Can you work these out from the model? Positions are in its coordinate system, mm. Face numbers are marked on the shaded views. A direction names the side the tool comes from. Give positions to 0.01 mm unless a question says otherwise; leave off trailing zeros. Loops run counter-clockwise (first coordinate to the right, second up) from the corner with the lowest first, then second, coordinate; pieces in that order, holes last. Notation, with made-up numbers: (-17.75, -27.75) - (-7.75, -27.75) arc R15 cw to (-7.75, -1.75) - close; hole circle Ø9 at (69, 66). An arc over 180 degrees is marked (long way). Use a Markdown table: item, result. Add a question column.
```python
from build123d import *

# Parameters (mm, degrees)
F0_W          = 25
F0_H          = 10
F1_DEPTH      = 4
F2_W          = 5
F2_H          = 10
F3_DEPTH      = 10
F4_R          = 1.25
F5_DEPTH      = 4.001
F7_R          = 4.99999
F8_R          = 1.55
F9_DEPTH      = 15.001
F10_R         = 1
F11_T1_DEPTH  = 8
F11_T6_ANGLE  = 233.2969892374
F11_T11_ANGLE = 233.2969892374
F11_T16_ANGLE = 233.2969892374
F11_T21_ANGLE = 233.2969892374


# Not quite as in the source:
# - a fillet or chamfer that OpenCascade refuses, or shapes differently, is made with other operations: its cross-section is extruded or revolved along the edge and cut away or added
# - a fillet or chamfer is up to 0.001 mm smaller than in the source, because OpenCascade refuses the exact size
# - a pattern or mirror of a feature is missing from the dataset's text; its kind, count and spacing are read off the source's solid


with BuildPart() as f1:
    # F0 (on Top) → F1 (new body)
    with BuildSketch(Plane.XY):
        Rectangle(F0_W, F0_H)
    extrude(amount=F1_DEPTH)

    # F2 (on face) → F3 (join)
    with BuildSketch(Plane.XY.offset(4)):
        Rectangle(F2_W, F2_H)
    extrude(amount=F3_DEPTH)

    # F4 (on face) → F5 (cut, through all)
    with BuildSketch(Plane.XY.offset(4)):
        with Locations((-7.5, 0)):
            Circle(F4_R)
    f5 = extrude(amount=-F5_DEPTH, mode=Mode.SUBTRACT)

    # F5_copies: F5 across plane
    add(f5.mirror(Plane(origin=(0, 0, 0), x_dir=(0, 0, 1), z_dir=(1, 0, 0))), mode=Mode.SUBTRACT)

    # F7 (radius 5 in the source; OpenCascade refuses exactly that, so slightly less here)
    f7_edges = [f1.edges().sort_by_distance(p)[0] for p in [
        (0, -5, 14),
        (0, 5, 14),
    ]]
    fillet(f7_edges, radius=F7_R)

    # F8 (on face) → F9 (cut, through all)
    with BuildSketch(Plane(origin=(-2.5, 0, 0), x_dir=(0, -1, 0), z_dir=(-1, 0, 0))):
        with Locations((0, 9)):
            Circle(F8_R)
    extrude(amount=-F9_DEPTH, mode=Mode.SUBTRACT)

    # F10
    f10_edges = [f1.edges().sort_by_distance(p)[0] for p in [
        (7.5, -5, 4),
        (12.5, 0, 4),
        (7.5, 5, 4),
        (12.5, -5, 2),
        (12.5, 5, 2),
        (-12.5, -5, 2),
        (-12.5, 5, 2),
        (-12.5, 0, 4),
        (-7.5, -5, 4),
        (-7.5, 5, 4),
    ]]
    fillet(f10_edges, radius=F10_R)

    # F11: fillet of radius 1 on 2 edges, made by hand

    # F11_s2 → F11_t1 (join)
    with BuildSketch(Plane.XZ.offset(-4)):
        with BuildLine():
            ThreePointArc((2.5, 5), (2.7928932188, 4.2928932188), (3.5, 4))
            Line((3.5, 4), (2.5, 4))
            Line((2.5, 4), (2.5, 5))
        make_face()
        with BuildLine():
            ThreePointArc((-2.5, 5), (-2.7928932188, 4.2928932188), (-3.5, 4))
            Line((-3.5, 4), (-2.5, 4))
            Line((-2.5, 4), (-2.5, 5))
        make_face()
    extrude(amount=F11_T1_DEPTH)


with BuildPart() as f11_tool4:
    # F11_s5 → F11_t6 (revolve)
    with BuildSketch(Plane.XZ.offset(-4)):
        with BuildLine():
            ThreePointArc((-2.5, 5), (-2.7928932188, 4.2928932188), (-3.5, 4))
            Line((-3.5, 4), (-2.5, 4))
            Line((-2.5, 4), (-2.5, 5))
        make_face()
    revolve(axis=Axis((-2.5, 4, 3), (-1, 0, 0)), revolution_arc=F11_T6_ANGLE)

    split(bisect_by=Plane.XZ.offset(-5), keep=Keep.TOP)


with BuildPart() as f1_1:
    add(f1.part)

    # F11_t3: union F11_tool4
    add(f11_tool4.part)


with BuildPart() as f11_tool9:
    # F11_s10 → F11_t11 (revolve)
    with BuildSketch(Plane(origin=(0, 0.0087041916, 0.0116762883), x_dir=(1, 0, 0), z_dir=(0, 0.5976672776, 0.8017442393))):
        with BuildLine():
            ThreePointArc((-3.5, -3.9999787901), (-2.7928932188, -3.7070855713), (-2.5, -2.9999787901))
            Line((-2.5, -2.9999787901), (-2.5, -3.9999787901))
            Line((-2.5, -3.9999787901), (-3.5, -3.9999787901))
        make_face()
    revolve(axis=Axis((-2.5, -4, 3), (-1, 0, 0)), revolution_arc=F11_T11_ANGLE)

    split(bisect_by=Plane.XZ.offset(5), keep=Keep.BOTTOM)


with BuildPart() as f1_2:
    add(f1_1.part)

    # F11_t8: union F11_tool9
    add(f11_tool9.part)


with BuildPart() as f11_tool14:
    # F11_s15 → F11_t16 (revolve)
    with BuildSketch(Plane(origin=(0, 0.0087041916, 0.0116762883), x_dir=(1, 0, 0), z_dir=(0, 0.5976672776, 0.8017442393))):
        with BuildLine():
            ThreePointArc((3.5, -3.9999787901), (2.7928932188, -3.7070855713), (2.5, -2.9999787901))
            Line((2.5, -2.9999787901), (2.5, -3.9999787901))
            Line((2.5, -3.9999787901), (3.5, -3.9999787901))
        make_face()
    revolve(axis=Axis((2.5, -4, 3), (-1, 0, 0)), revolution_arc=F11_T16_ANGLE)

    split(bisect_by=Plane.XZ.offset(5), keep=Keep.BOTTOM)


with BuildPart() as f1_3:
    add(f1_2.part)

    # F11_t13: union F11_tool14
    add(f11_tool14.part)


with BuildPart() as f11_tool19:
    # F11_s20 → F11_t21 (revolve)
    with BuildSketch(Plane.XZ.offset(-4)):
        with BuildLine():
            ThreePointArc((2.5, 5), (2.7928932188, 4.2928932188), (3.5, 4))
            Line((3.5, 4), (2.5, 4))
            Line((2.5, 4), (2.5, 5))
        make_face()
    revolve(axis=Axis((2.5, 4, 3), (-1, 0, 0)), revolution_arc=F11_T21_ANGLE)

    split(bisect_by=Plane.XZ.offset(-5), keep=Keep.TOP)


with BuildPart() as f1_4:
    add(f1_3.part)

    # F11_t18: union F11_tool19
    add(f11_tool19.part)


solid = f1_4.part
```
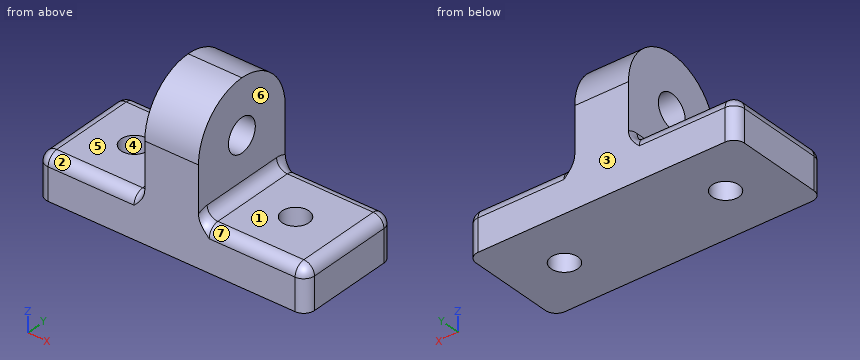
1. Will these pins go through, and if not, where does the flat tip stop? P1, Ø1.9, axis at y = 0, z = 9, coming from the -X side; P2, Ø3, axis at y = -2, z = 9.5, coming from the +X side; P3, Ø3, axis at x = 3.5, y = -2, coming from the +Z side; P4, Ø4, axis at x = -7.5, y = 0, coming from the +Z side.
2. If we mould it in two halves opening along Y, with no side actions, what happens to the marked faces 1, 2, 3 and 4? For each: released by +Y, released by -Y, zero draft, split by the parting line, or undercut.
3. Suppose I cut it at B-B (z = 7.75). List the corners of the cut face in (x, y) for me, and give its area (3 significant figures).
4. Please list where these lines run through material, in increasing order: line 1 along Z through (x, y) = (-0.95, 0); line 2 along Z through (x, y) = (-10.25, 0.75); line 3 along X through (y, z) = (1, 11.75). Write a range as [from, to].
5. Suppose I cut it at D-D (z = 2.5). List the corners of the cut face in (x, y) for me.
6. Suppose I cut it at C-C (x = 7.5). List the corners of the cut face in (y, z) for me, and give its area (3 significant figures).
7. On a 3-axis mill with a long thin cutter (end or side, diameter ignored), from which of +Z, -Z, +X, -X, +Y, -Y can I reach the whole of each face in a straight line? I mean the marked faces 5, 6 and 7. Say none if no direction works.
Results below:
| question | item | result |
|---|---|---|
| 1 | P1 | through |
| 1 | P2 | x = 2.5 |
| 1 | P3 | z = 13.92 |
| 1 | P4 | z = 4 |
| 2 | face 1 | zero draft |
| 2 | face 2 | released by -Y |
| 2 | face 3 | released by +Y |
| 2 | face 4 | undercut |
| 3 | outline | (-2.5, -5) - (2.5, -5) - (2.5, -0.92) - (-2.5, -0.92) - close; (-2.5, 0.92) - (2.5, 0.92) - (2.5, 5) - (-2.5, 5) - close |
| 3 | area | 40.8 mm² |
| 4 | line 1 | [0, 7.45], [10.55, 14] |
| 4 | line 2 | [0, 4] |
| 4 | line 3 | [-2.5, 2.5] |
| 5 | outline | (-12.5, -4) arc R1 ccw to (-11.5, -5) - (11.5, -5) arc R1 ccw to (12.5, -4) - (12.5, 4) arc R1 ccw to (11.5, 5) - (-11.5, 5) arc R1 ccw to (-12.5, 4) - close; hole circle Ø2.5 at (-7.5, 0); hole circle Ø2.5 at (7.5, 0) |
| 6 | outline | (-5, 0) - (-1.25, 0) - (-1.25, 4) - (-4, 4) arc R1 ccw to (-5, 3) - close; (1.25, 0) - (5, 0) - (5, 3) arc R1 ccw to (4, 4) - (1.25, 4) - close |
| 6 | area | 29.6 mm² |
| 7 | face 5 | +Z, -X, +Y, -Y |
| 7 | face 6 | +Z, +X, +Y, -Y |
| 7 | face 7 | +Z, +X, -Y |
